from build123d import *

# Parameters (mm, degrees)
ESBO_O1_R          = 4
ESBO_O1_R_2        = 5
FLANGE_BASE1_DEPTH = 3


# Sheet-metal steps are written as plain solids
with BuildPart() as part:
    # Esboço1 → Flange-base1 (new body)
    with BuildSketch(Plane(origin=(0, 0, 0), x_dir=(1, 0, 0), z_dir=(0, 1, 0))):
        with BuildLine():
            Line((0, 0), (0, 50))
            Line((0, 50), (60, 50))
            Line((60, 50), (60, 0))
            ThreePointArc((60, 0), (54.142135624, -14.142135624), (40, -20))
            Line((40, -20), (20, -20))
            ThreePointArc((20, -20), (5.857864376, -14.142135624), (0, 0))
        make_face()
        with Locations(Location((30, -10, 0), (0, 0, 270))):
            Circle(ESBO_O1_R, mode=Mode.SUBTRACT)
        with Locations(Location((18.029294984, -7.889241728, 0), (0, 0, 270))):
            Circle(ESBO_O1_R, mode=Mode.SUBTRACT)
        with Locations(Location((7.502433661, -1.811555509, 0), (0, 0, 270))):
            Circle(ESBO_O1_R, mode=Mode.SUBTRACT)
        with Locations(Location((52.497566339, -1.811555509, 0), (0, 0, 90))):
            Circle(ESBO_O1_R, mode=Mode.SUBTRACT)
        with Locations(Location((41.970705016, -7.889241728, 0), (0, 0, 90))):
            Circle(ESBO_O1_R, mode=Mode.SUBTRACT)
        with Locations(Location((30, 25, 0), (0, 0, 270))):
            Circle(ESBO_O1_R_2, mode=Mode.SUBTRACT)
    extrude(amount=-FLANGE_BASE1_DEPTH)


solid = part.part
The listing builds one solid part. Answer for the finished solid, in the listing's coordinates (mm). Give positions to 0.01 mm unless a question says otherwise; leave off trailing zeros. Write each loop counter-clockwise with the first axis right and the second up, starting at its lowest first coordinate (ties: lowest second). Pieces come first, ordered by that corner, then holes.
1) Section B-B (z = -29) is taken. Write down the section's boundary in (x, y), and give its area (3 significant figures).
2) Given P1, Ø7, axis at x = 18.03, z = 7.89, coming from the +Y side; P2, Ø1, axis at x = 46, y = -0.5, coming from the +Z side, each flat-ended and moving along its own axis, determine where each tip first touches the part or whether it passes through.
3) Section D-D (x = 6.5) is taken. Write down the section's boundary in (y, z), and give its area (3 significant figures).
4) Find the intervals of material crossed by L1, parallel to Z at x = 28, y = -2.7; L2, parallel to X at y = -0.75, z = 10; L3, parallel to X at y = -2.2, z = 7 (3 decimals), in increasing order.
5) For a pull along X with two mould halves and no side action, classify faces 1 (the face through (30, 0, -15)), 2 (the face through (38.005, -1.479, 8.41)), 3 (the face through (60, -1, -25)) as pulls with the +X half, pulls with the -X half, needs draft (parallel to the pull), parting line crosses it, or undercut.
6) Section A-A (x = 30) is taken. Write down the section's boundary in (y, z), and give its area (3 significant figures).
7) Section C-C (z = 5) is taken. Write down the section's boundary in (x, y), and give its area (3 significant figures).
Response:
1. outline: (0, -3) - (27, -3) - (27, 0) - (0, 0) - close; (33, -3) - (60, -3) - (60, 0) - (33, 0) - close
1. area: 162 mm2
2. P1: passes through
2. P2: stops at z = 19.23
3. outline: (-3, -50) - (0, -50) - (0, -2.06) - (-3, -2.06) - close; (-3, 5.68) - (0, 5.68) - (0, 14.76) - (-3, 14.76) - close
3. area: 171 mm2
4. L1: z = -50 to -29.58, -20.42 to 6.54, 13.46 to 20
4. L2: x = 2.68 to 14.63, 21.43 to 26, 34 to 38.57, 45.37 to 57.32
4. L3: x = 1.265 to 14.129, 21.929 to 27.354, 32.646 to 38.071, 45.871 to 58.735
5. face 1: needs draft
5. face 2: undercut
5. face 3: pulls with the +X half
6. outline: (-3, -50) - (0, -50) - (0, -30) - (-3, -30) - close; (-3, -20) - (0, -20) - (0, 6) - (-3, 6) - close; (-3, 14) - (0, 14) - (0, 20) - (-3, 20) - close
6. area: 156 mm2
7. outline: (0.64, -3) - (5.09, -3) - (5.09, 0) - (0.64, 0) - close; (9.92, -3) - (15.26, -3) - (15.26, 0) - (9.92, 0) - close; (20.8, -3) - (39.2, -3) - (39.2, 0) - (20.8, 0) - close; (44.74, -3) - (50.08, -3) - (50.08, 0) - (44.74, 0) - close; (54.91, -3) - (59.36, -3) - (59.36, 0) - (54.91, 0) - close
7. area: 114 mm2
